from build123d import *

# Parameters (mm, degrees)
SKETCH1_W           = 250
SKETCH1_H           = 50
BOSS_EXTRUDE1_DEPTH = 10
FILLET2_R           = 25
SKETCH4_R           = 6.75
CUT_EXTRUDE3_DEPTH  = 128.867118525
SKETCH5_W           = 110
SKETCH5_H           = 10
BOSS_EXTRUDE2_DEPTH = 20
SKETCH6_W           = 50
SKETCH6_H           = 10
BOSS_EXTRUDE3_DEPTH = 20
FILLET3_R           = 10
FILLET4_R           = 5
SKETCH7_R           = 2.5527
CUT_EXTRUDE4_DEPTH  = 134.229125945


with BuildPart() as part:
    # Sketch1 → Boss-Extrude1 (new body)
    with BuildSketch(Plane(origin=(0, 0, 0), x_dir=(1, 0, 0), z_dir=(0, 1, 0))):
        Rectangle(SKETCH1_W, SKETCH1_H)
    extrude(amount=BOSS_EXTRUDE1_DEPTH)

    # Fillet2
    fillet2_edges = [part.edges().sort_by_distance(p)[0] for p in [
        (-125, 5, 25),
        (-125, 5, -25),
    ]]
    fillet(fillet2_edges, radius=FILLET2_R - 0.0001)  # a hair under: the kernel refuses the full size

    # Sketch4 → Cut-Extrude3 (cut, through all)
    with BuildSketch(Plane(origin=(0, 10, 0), x_dir=(1, 0, 0), z_dir=(0, 1, 0))):
        with Locations(Location((-100, 0, 0), (0, 0, 270))):
            Circle(SKETCH4_R)
    extrude(amount=-CUT_EXTRUDE3_DEPTH, mode=Mode.SUBTRACT)

    # Sketch5 → Boss-Extrude2 (add)
    with BuildSketch(Plane(origin=(0, 0, -25), x_dir=(-1, 0, 0), z_dir=(0, 0, -1))):
        with Locations((-70, 5)):
            Rectangle(SKETCH5_W, SKETCH5_H)
    extrude(amount=BOSS_EXTRUDE2_DEPTH)

    # Sketch6 → Boss-Extrude3 (add)
    with BuildSketch(Plane.XY.offset(25)):
        with Locations((100, 5)):
            Rectangle(SKETCH6_W, SKETCH6_H)
    extrude(amount=BOSS_EXTRUDE3_DEPTH)

    # Fillet3
    fillet3_edges = [part.edges().sort_by_distance(p)[0] for p in [
        (15, 5, -25),
        (75, 5, 25),
    ]]
    fillet(fillet3_edges, radius=FILLET3_R)

    # Fillet4
    fillet4_edges = [part.edges().sort_by_distance(p)[0] for p in [
        (125, 5, -45),
        (15, 5, -45),
    ]]
    fillet(fillet4_edges, radius=FILLET4_R)

    # Sketch7 → Cut-Extrude4 (cut, through all)
    with BuildSketch(Plane.XZ):
        with Locations(Location((70, -25, 0), (0, 0, 270))):
            Circle(SKETCH7_R)
    extrude(amount=-CUT_EXTRUDE4_DEPTH, mode=Mode.SUBTRACT)


solid = part.part
Model file for the job. Use its own axes, mm. A direction names the side the tool comes from. Round coordinates to 2 decimals unless told otherwise and drop trailing zeros. Loops run counter-clockwise (first coordinate to the right, second up) from the corner with the lowest first, then second, coordinate; pieces in that order, holes last.
1. Mould opens along X. For faces 4 (the cylindrical face through (-95.438, 5.07, -4.975)), 5 (the cylindrical face through (-117.871, 5.07, -17.482)), 6 (the cylindrical face through (67.735, 4.93, -26.178)), 7 (the flat face through (125, 5, 2)) say: +X half, -X half, draft (parallel to the pull), parting line (faces both ways), or undercut.
Check values:
face 4: undercut
face 5: -X half
face 6: undercut
face 7: +X half
2. Band-saw the part on C-C, the plane x = -39. List the corners of the cut face in (y, z).
Check values:
outline: (0, -25) - (10, -25) - (10, 25) - (0, 25) - close
3. Wall check: probe 1 along Z at (x, y) = (-73, 1); probe 2 along X at (y, z) = (2.5, 0); probe 3 along Z at (x, y) = (49, 6.75). Give the ranges that are in metal, low to high.
Check values:
probe 1: z = -25 to 25
probe 2: x = -125 to -106.75, -93.25 to 125
probe 3: z = -45 to 25
4. Tool access for faces 1 (the flat face through (15, 5, -37)), 2 (the flat face through (26, 0, -1)), 3 (the flat face through (-19, 5, 25)): list every direction of +Z, -Z, +X, -X, +Y, -Y with a clear straight run to the whole face (end or side of a thin tool).
Check values:
face 1: -Z, -X, +Y, -Y
face 2: +Z, -Z, +X, -X, -Y
face 3: +Z, -X, +Y, -Y
5. Band-saw the part on B-B, the plane x = 70. List the corners of the cut face in (y, z), and give its area (3 significant figures).
Check values:
outline: (0, -45) - (10, -45) - (10, -27.55) - (0, -27.55) - close; (0, -22.45) - (10, -22.45) - (10, 26.34) - (0, 26.34) - close
area: 662 mm2
6. Band-saw the part on A-A, the plane y = 7.25. Count the separate pieces of the cut face and the enclosed holes in it, and give its area (3 significant figures).
Check values:
separate pieces: 1
enclosed holes: 2
area: 15,300 mm2
7. Band-saw the part on D-D, the plane x = 17.5. List the corners of the cut face in (y, z).
Check values:
outline: (0, -44.33) - (10, -44.33) - (10, 25) - (0, 25) - close
8. Drop flat-ended pins along their axis: P1, Ø5.5, axis at y = 3, z = -38, coming from the -X side; P2, Ø12, axis at x = -30.5, z = -34.5, coming from the +Y side; P3, Ø4, axis at y = 9, z = -3.5, coming from the -X side; P4, Ø3, axis at x = -40, y = 3, coming from the -Z side. Give the stop position or say it passes through.
Check values:
P1: stops at x = 15
P2: passes through
P3: stops at x = -124.95
P4: stops at z = -25
